Input: part model. Units: mm. Frame: model coordinates. Face numbers are marked on the shaded views. A direction names the side the tool comes from. Round coordinates to 2 decimals unless told otherwise and drop trailing zeros. Loops run counter-clockwise (first coordinate to the right, second up) from the corner with the lowest first, then second, coordinate; pieces in that order, holes last. Notation, with made-up numbers: (55.25, 23.25) -> (76.25, 23.25) arc R21 cw to (76.25, 31.25) -> close; hole circle Ø4 at (77.25, 82). An arc over 180 degrees is marked (long way). Answer in a Markdown table with one row per item. Add a question column.
Q1. Pin query (flat end, axial travel): pin 1 (19 mm diameter, centred on y = 10, z = 35, fed in from -X); pin 2 (1 mm diameter, centred on x = -28, z = 39, fed in from +Y); pin 3 (16 mm diameter, centred on y = 14, z = 30, fed in from +X). Return the tip coordinate at first contact, or that it passes through.
Q2. Reachability of the marked faces 1, 2 and 3 from +Z, -Z, +X, -X, +Y, -Y: full face, straight path, thin tool, end or side. Return the list, or none.
Q3. Mould query, pull axis Z, two halves, no side actions, for the marked faces 4, 5, 6 and 7. Classes: pulls with the +Z half, pulls with the -Z half, needs draft (parallel to the pull), parting line crosses it, or undercut.
Q4. Section D-D, the plane y = -10. Output: boundary loops of the cut face in (x, z), and give its area (3 significant figures).
Q5. Section A-A, the plane x = 40. Output: boundary loops of the cut face in (y, z), and give its area (3 significant figures).
Q6. Ray query, L1, parallel to Z at x = -14, y = 18; L2, parallel to Z at x = 10, y = -5; L3, parallel to X at y = 15.5, z = 48.5. Return the intervals inside material, ascending. Write a range as from..to.
Q7. Section C-C, the plane z = 47. Output: boundary loops of the cut face in (x, y).
Q8. Section B-B, the plane y = 10. Output: boundary loops of the cut face in (x, z).
```python
from build123d import *

# Parameters (mm, degrees)
EXTRUDE_1_DEPTH     = 70
SKETCH_2_W          = 84
SKETCH_2_H          = 54
CUT_EXTRUDE_1_DEPTH = 20
SKETCH_3_R          = 7.5
CUT_EXTRUDE_2_DEPTH = 89.317608663
CUT_EXTRUDE_3_DEPTH = 89.317608663
SKETCH_4_R          = 6
CUT_EXTRUDE_4_DEPTH = 118.320075008


with BuildPart() as part:
    # Эскиз1 → Бобышка-Вытянуть1 (new body)
    with BuildSketch(Plane.XY):
        Polygon((50, -20), (50, 0), (20, 0), (-10, 20), (-50, 20), (-50, -20), align=None)
    extrude(amount=EXTRUDE_1_DEPTH)

    # Эскиз2 → Вырез-Вытянуть1 (cut)
    with BuildSketch(Plane(origin=(0, 20, 0), x_dir=(1, 0, 0), z_dir=(0, 1, 0))):
        with Locations((0, -35)):
            Rectangle(SKETCH_2_W, SKETCH_2_H)
    extrude(amount=-CUT_EXTRUDE_1_DEPTH, mode=Mode.SUBTRACT)

    # Эскиз3 → Вырез-Вытянуть2 (cut, through all)
    with BuildSketch(Plane(origin=(0, 0, 0), x_dir=(1, 0, 0), z_dir=(0, 1, 0))):
        with Locations(Location((10, -35, 0), (0, 0, 180))):
            Circle(SKETCH_3_R)
    extrude(amount=-CUT_EXTRUDE_2_DEPTH, mode=Mode.SUBTRACT)

    # Эскиз3<4> → Вырез-Вытянуть3 (cut, through all)
    with BuildSketch(Plane(origin=(0, 0, 0), x_dir=(1, 0, 0), z_dir=(0, 1, 0))):
        with BuildLine():
            Line((35, -20), (35, -15))
            ThreePointArc((35, -15), (40, -10), (45, -15))
            Line((45, -15), (45, -20))
            ThreePointArc((45, -20), (40, -25), (35, -20))
        make_face()
    cut_extrude_3 = extrude(amount=-CUT_EXTRUDE_3_DEPTH, mode=Mode.SUBTRACT)

    # Зеркальное отражение1: Вырез-Вытянуть3 across plane
    add(cut_extrude_3.mirror(Plane(origin=(0, 0, 35), x_dir=(1, 0, 0), z_dir=(0, 0, -1))), mode=Mode.SUBTRACT)

    # Эскиз4 → Вырез-Вытянуть4 (cut, through all)
    with BuildSketch(Plane(origin=(-42, 0, 0), x_dir=(0, 0, -1), z_dir=(1, 0, 0))):
        with Locations(Location((-35, 10, 0), (0, 0, 90))):
            Circle(SKETCH_4_R)
    extrude(amount=-CUT_EXTRUDE_4_DEPTH, mode=Mode.SUBTRACT)


solid = part.part
```
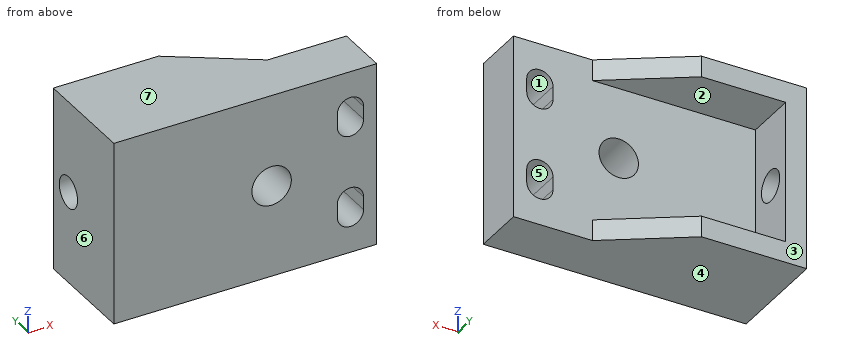
Answer block:
| question | item | result |
|---|---|---|
| 1 | pin 1 | x = -50 |
| 1 | pin 2 | y = 0 |
| 1 | pin 3 | x = -42 |
| 2 | face 1 | +Y, -Y |
| 2 | face 2 | +X, +Y |
| 2 | face 3 | +Z, -Z, +X, -X, +Y |
| 3 | face 4 | pulls with the -Z half |
| 3 | face 5 | undercut |
| 3 | face 6 | needs draft |
| 3 | face 7 | pulls with the +Z half |
| 4 | outline | (-50, 0) -> (50, 0) -> (50, 70) -> (-50, 70) -> close; hole circle Ø15 at (10, 35); hole (35, 15) arc R5 ccw to (45, 15) -> (45, 20) arc R5 ccw to (35, 20) -> close; hole (35, 50) arc R5 ccw to (45, 50) -> (45, 55) arc R5 ccw to (35, 55) -> close |
| 4 | area | 6,570 mm^2 |
| 5 | outline | (-20, 0) -> (0, 0) -> (0, 10) -> (-20, 10) -> close; (-20, 25) -> (0, 25) -> (0, 45) -> (-20, 45) -> close; (-20, 60) -> (0, 60) -> (0, 70) -> (-20, 70) -> close |
| 5 | area | 800 mm^2 |
| 6 | L1 | 0..8, 62..70 |
| 6 | L2 | 0..27.5, 42.5..70 |
| 6 | L3 | -50..-42 |
| 7 | outline | (-50, -20) -> (36, -20) -> (36, 0) -> (-42, 0) -> (-42, 20) -> (-50, 20) -> close; (44, -20) -> (50, -20) -> (50, 0) -> (44, 0) -> close |
| 8 | outline | (-50, 0) -> (5, 0) -> (5, 8) -> (-42, 8) -> (-42, 29) -> (-50, 29) -> close; (-50, 41) -> (-42, 41) -> (-42, 62) -> (5, 62) -> (5, 70) -> (-50, 70) -> close |
